```python
from build123d import *

# Parameters (mm, degrees)
F0_R     = 15.24
F1_DEPTH = 25


# Not quite as in the source:
# - a feature names something its author has since deleted; it is built from what else it names


with BuildPart() as f1:
    # F0 (on Front) → F1 (new body)
    with BuildSketch(Plane.XZ):
        with BuildLine():
            ThreePointArc((17.3446724068, 18.5559246361), (23.2992991218, 10.1144777637), (25.4, 0))
            ThreePointArc((25.4, 0), (23.2992991218, -10.1144777637), (17.3446724068, -18.5559246361))
            Line((17.3446724068, -18.5559246361), (116.5943626679, -15.9569800311))
            ThreePointArc((116.5943626679, -15.9569800311), (107.95, 0), (116.5943626679, 15.9569800311))
            Line((116.5943626679, 15.9569800311), (17.3446724068, 18.5559246361))
        make_face()
        with BuildLine():
            ThreePointArc((17.3446724068, -18.5559246361), (23.2992991218, -10.1144777637), (25.4, 0))
            ThreePointArc((25.4, 0), (23.2992991218, 10.1144777637), (17.3446724068, 18.5559246361))
            ThreePointArc((17.3446724068, 18.5559246361), (-25.4, 0), (17.3446724068, -18.5559246361))
        make_face()
        Circle(F0_R, mode=Mode.SUBTRACT)
        with BuildLine():
            ThreePointArc((146.05, 0), (136.0740043207, 16.7500730025), (116.5943626679, 15.9569800311))
            ThreePointArc((116.5943626679, 15.9569800311), (107.95, 0), (116.5943626679, -15.9569800311))
            ThreePointArc((116.5943626679, -15.9569800311), (136.0740043207, -16.7500730025), (146.05, 0))
        make_face()
        with Locations((127, 0)):
            Circle(F0_R, mode=Mode.SUBTRACT)
    extrude(amount=F1_DEPTH)


solid = f1.part
```
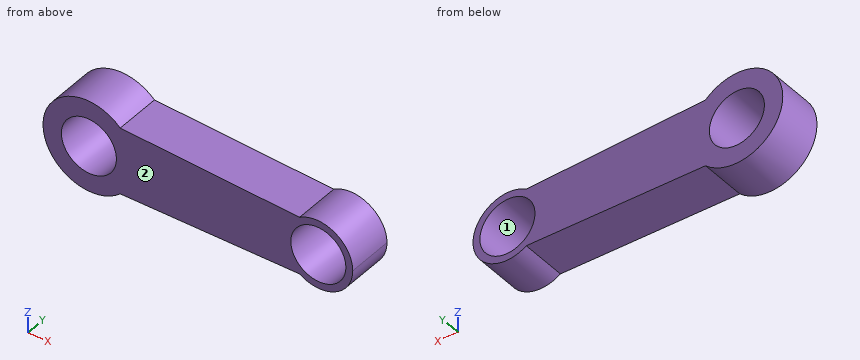
CAD build for the part. Positions are in the model's coordinates, mm. Face numbers are marked on the shaded views. Give positions to 0.01 mm unless a question says otherwise; leave off trailing zeros. Order: outer loops, then holes, each group sorted by start corner. A loop starts at its lowest first (then second) coordinate and runs counter-clockwise, first axis right, second up. Notation, with made-up numbers: M 1,2 L 21,2 A29 cw 21,23 Z; hole C 65.25,15.25 d3. An arc over 180 degrees is marked long. Put each result on its own line as item: value. Start each with the question number.
(1) Saw through at A-A, the plane x = 0. Write the cut outline in (y, z), then the cut area to 3 significant figures.
(2) Saw through at D-D, the plane x = 127. Write the cut outline in (y, z), then the cut area to 4 significant figures.
(3) Drill centre lines: line 1 along X through (y, z) = (-16.25, 7); line 2 along Z through (x, y) = (0, -11.25); line 3 along X through (y, z) = (-23.5, 6). Where is each one in solid material? Low to high.
(4) Flat gauge pins, fed straight in: pin 1 Ø2 at (x, z) = (50, -2) entering from +Y; pin 2 Ø18.5 at (x, z) = (127, 0) entering from -Y; pin 3 Ø6 at (x, y) = (81, -15) entering from -Z; pin 4 Ø12 at (x, y) = (75.5, -22) entering from +Z. Where does each tip first touch, or does it go through?
(5) Saw through at B-B, the plane y = -12.5. Write the cut outline in (x, z), then the cut area to 3 significant figures.
(6) Mould opens along X. For the marked faces 1 and 2 say: +X half, -X half, draft (parallel to the pull), parting line (faces both ways), or undercut.
(7) Saw through at C-C, the plane z = -13. Write the cut outline in (x, y).
Check result:
1. outline: M -25,-25.4 L 0,-25.4 L 0,-15.24 L -25,-15.24 Z; M -25,15.24 L 0,15.24 L 0,25.4 L -25,25.4 Z
1. area: 508 mm2
2. outline: M -25,-19.05 L 0,-19.05 L 0,-15.24 L -25,-15.24 Z; M -25,15.24 L 0,15.24 L 0,19.05 L -25,19.05 Z
2. area: 190.5 mm2
3. line 1: x = -24.42 to -13.54, 13.54 to 113.46, 140.54 to 144.72
3. line 2: z = -25.4 to -15.24, 15.24 to 25.4
3. line 3: x = -24.68 to -14.01, 14.01 to 112.99, 141.01 to 145.08
4. pin 1: stops at y = 0
4. pin 2: passes through
4. pin 3: stops at z = -16.97
4. pin 4: stops at z = 17.19
5. outline: M 17.34,-18.56 L 116.59,-15.96 A19.05 ccw long 116.59,15.96 L 17.34,18.56 A25.4 ccw long Z; hole C 0,0 d30.48; hole C 127,0 d30.48
5. area: 4,730 mm2
6. face 1: undercut
6. face 2: draft
7. outline: M -21.82,-25 L -7.95,-25 L -7.95,0 L -21.82,0 Z; M 7.95,-25 L 119.05,-25 L 119.05,0 L 7.95,0 Z; M 134.95,-25 L 140.92,-25 L 140.92,0 L 134.95,0 Z
